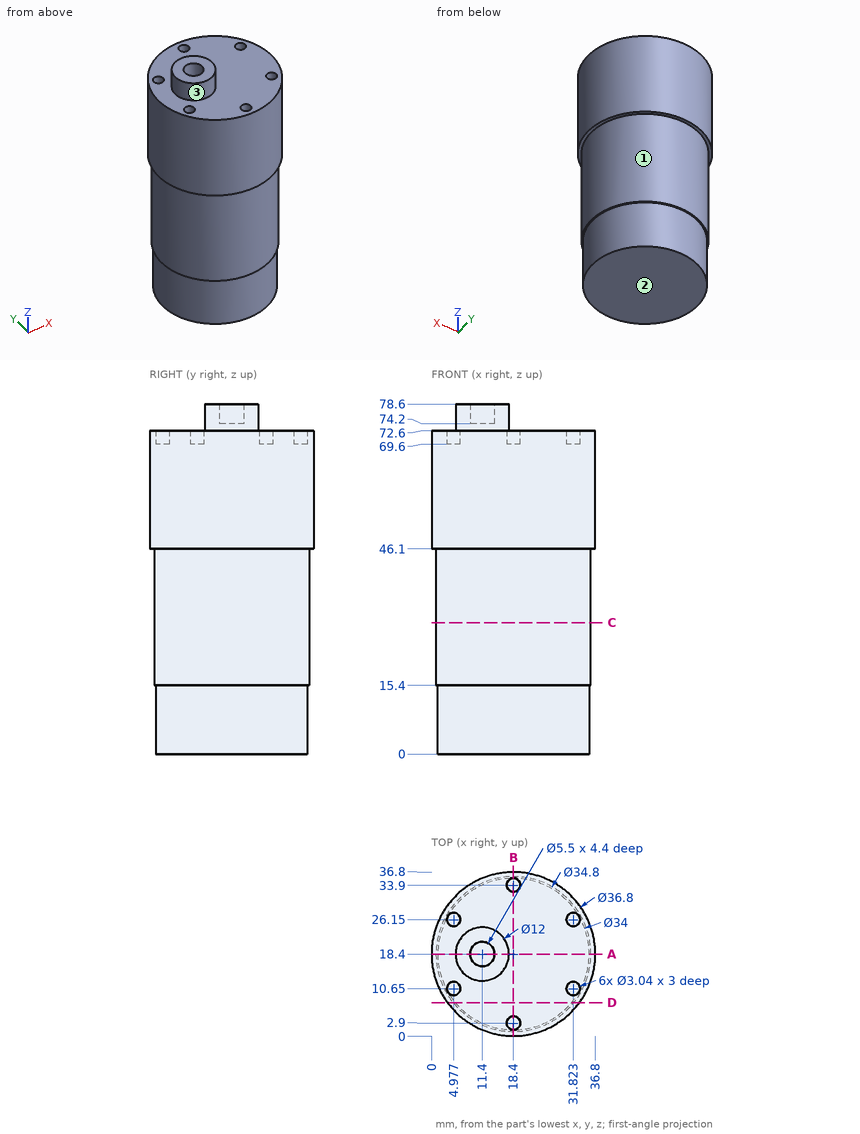
Input: dimensioned drawing with shaded views. Units: mm. Origin: part minimum x, y, z. A direction names the side the tool comes from. Give positions to 0.01 mm unless a question says otherwise; leave off trailing zeros. Loops run counter-clockwise (first coordinate to the right, second up) from the corner with the lowest first, then second, coordinate; pieces in that order, holes last. Notation, with made-up numbers: M -37.5,-15 L -16.5,-15 A24 ccw -16.5,24 Z; hole C -26,87.25 d9. An arc over 180 degrees is marked long. Put each result on its own line as item: value. Start each with the question number.
1) Access query for the marked faces 1, 2 and 3. Directions: +Z, -Z, +X, -X, +Y, -Y. A direction counts if a zero-diameter tool reaches every point of the face in a straight line with its end or side. Return the directions, or none.
2) Cut plane D-D (y = 7.5). Output: boundary loops of the cut face in (x, z) (1 decimal).
3) Cut plane B-B (x = 18.4). Output: boundary loops of the cut face in (y, z), then the cut area to 3 significant figures.
4) Ray query, line 1 along Z through (x, y) = (16.5, 28.5); line 2 along X through (y, z) = (22, 21.5); line 3 along Z through (x, y) = (9.5, 19.5). Return the intervals inside material, ascending.
5) Contact query for flat-ended pins moving along their axis: pin 1 (1.8 mm diameter, centred on x = 18.4, y = 2.9, fed in from -Z); pin 2 (0.9 mm diameter, centred on x = 4.5, y = 10, fed in from +Z); pin 3 (3.5 mm diameter, centred on x = 19, y = 34, fed in from +Z); pin 4 (1.5 mm diameter, centred on y = 14, z = 46.5, fed in from +X) (1 decimal). Output: stop coordinate, or through.
6) Cut plane A-A (y = 18.4). Output: boundary loops of the cut face in (x, z).
7) Cut plane C-C (z = 29.5). Output: boundary loops of the cut face in (x, y), then the cut area to 3 significant figures.
Verdict:
1. face 1: -Z
1. face 2: -Z, +X, -X, +Y, -Y
1. face 3: +Z
2. outline: M 3.6,46.1 L 4.8,46.1 L 4.8,15.4 L 5.4,15.4 L 5.4,0 L 31.4,0 L 31.4,15.4 L 32,15.4 L 32,46.1 L 33.2,46.1 L 33.2,72.6 L 3.6,72.6 Z
3. outline: M 0,46.1 L 1,46.1 L 1,15.4 L 1.4,15.4 L 1.4,0 L 35.4,0 L 35.4,15.4 L 35.8,15.4 L 35.8,46.1 L 36.8,46.1 L 36.8,72.6 L 35.42,72.6 L 35.42,69.6 L 32.38,69.6 L 32.38,72.6 L 4.42,72.6 L 4.42,69.6 L 1.38,69.6 L 1.38,72.6 L 0,72.6 Z
3. area: 2,550 mm2
4. line 1: 0 to 72.6
4. line 2: 1.38 to 35.42
4. line 3: 0 to 74.2
5. pin 1: z = 0
5. pin 2: z = 69.6
5. pin 3: z = 72.6
5. pin 4: x = 36.4
6. outline: M 0,46.1 L 1,46.1 L 1,15.4 L 1.4,15.4 L 1.4,0 L 35.4,0 L 35.4,15.4 L 35.8,15.4 L 35.8,46.1 L 36.8,46.1 L 36.8,72.6 L 17.4,72.6 L 17.4,78.6 L 14.15,78.6 L 14.15,74.2 L 8.65,74.2 L 8.65,78.6 L 5.4,78.6 L 5.4,72.6 L 0,72.6 Z
7. outline: C 18.4,18.4 d34.8
7. area: 951 mm2
